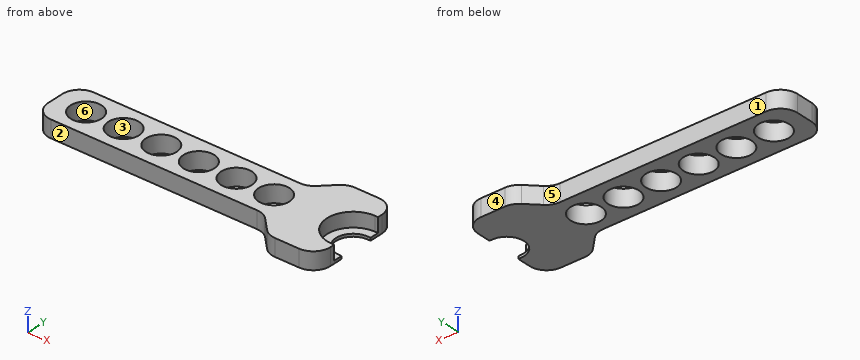
from build123d import *

# Parameters (mm, degrees)
F1_DEPTH    = 6.35
F3_DEPTH    = 5.334
F4_W        = 17.78
F4_H        = 8.255
F5_DEPTH    = 25.4
F6_R        = 5.715
F7_DEPTH    = 25.4
F8_T4_DEPTH = 6.35
F8_T9_DEPTH = 6.35
F9_R        = 6.35


# Not quite as in the source:
# - a fillet or chamfer that OpenCascade refuses, or shapes differently, is made with other operations: its cross-section is extruded or revolved along the edge and cut away or added


with BuildPart() as f1:
    # F0 (on Top) → F1 (new body)
    with BuildSketch(Plane.XY):
        Polygon((8.1444730278, -17.78), (17.78, -17.78), (17.78, 17.78), (-17.78, 17.78), (-17.78, 9.525), (-93.98, 9.525), (-93.98, -9.525), (-17.78, -9.525), (-17.78, -17.78), (-8.1444730278, -17.78), align=None)
    extrude(amount=F1_DEPTH)

    # F2 (on face) → F3 (cut)
    with BuildSketch(Plane.XY.offset(6.35)):
        with BuildLine():
            Line((17.78, 9.7409), (16.7259, 9.7409))
            ThreePointArc((16.7259, 9.7409), (6.985, 0), (16.7259, -9.7409))
            Line((16.7259, -9.7409), (17.78, -9.7409))
            Line((17.78, -9.7409), (17.78, 9.7409))
        make_face()
    extrude(amount=-F3_DEPTH, mode=Mode.SUBTRACT)

    # F4 (on face) → F5 (cut)
    with BuildSketch(Plane(origin=(0, 0, 0), x_dir=(1, 0, 0), z_dir=(0, 0, -1))):
        with BuildLine():
            Line((17.78, 6.4135), (16.7005, 6.4135))
            ThreePointArc((16.7005, 6.4135), (10.287, 0), (16.7005, -6.4135))
            Line((16.7005, -6.4135), (17.78, -6.4135))
            Line((17.78, -6.4135), (17.78, 6.4135))
        make_face()
        with Locations((-8.89, -13.6525)):
            Rectangle(F4_W, F4_H)
        with Locations((-8.89, 13.6525)):
            Rectangle(F4_W, F4_H)
    extrude(amount=-F5_DEPTH, mode=Mode.SUBTRACT)

    # F6 (on face) → F7 (cut)
    with BuildSketch(Plane.XY.offset(6.35)):
        with Locations((-82.55, 0)):
            Circle(F6_R)
        with Locations((-68.58, 0)):
            Circle(F6_R)
        with Locations((-54.61, 0)):
            Circle(F6_R)
        with Locations((-40.64, 0)):
            Circle(F6_R)
        with Locations((-26.67, 0)):
            Circle(F6_R)
        with Locations((-12.7, 0)):
            Circle(F6_R)
    extrude(amount=-F7_DEPTH, mode=Mode.SUBTRACT)

    # F8: chamfer of 8.382 on 2 edges, made by hand


with BuildPart() as f8_tool2:
    # F8_s3 → F8_t4 (new body)
    with BuildSketch(Plane.XY):
        Polygon((0, -17.907), (-8.382, -9.525), (0, -9.525), align=None)
    extrude(amount=F8_T4_DEPTH)

    split(bisect_by=Plane.XZ.offset(17.78), keep=Keep.BOTTOM)


with BuildPart() as f1_1:
    add(f1.part)

    # F8_t1: union F8_tool2
    add(f8_tool2.part)


with BuildPart() as f8_tool7:
    # F8_s8 → F8_t9 (new body)
    with BuildSketch(Plane.XY):
        Polygon((-8.382, 9.525), (0, 17.907), (0, 9.525), align=None)
    extrude(amount=F8_T9_DEPTH)

    split(bisect_by=Plane.XZ.offset(-17.78), keep=Keep.TOP)


with BuildPart() as f1_2:
    add(f1_1.part)

    # F8_t6: union F8_tool7
    add(f8_tool7.part)

    # F9
    f9_edges = [f1_2.edges().sort_by_distance(p)[0] for p in [
        (-8.382, -9.525, 3.175),
        (-8.382, 9.525, 3.175),
        (-0.127, 17.78, 3.175),
        (-0.127, -17.78, 3.175),
        (-93.98, 9.525, 3.175),
        (-93.98, -9.525, 3.175),
        (17.78, 17.78, 3.175),
        (17.78, -17.78, 3.175),
    ]]
    fillet(f9_edges, radius=F9_R)


solid = f1_2.part
Read the model definition and answer for the solid it produces. Units are mm, in the model's axes. Face numbers are marked on the shaded views. A direction names the side the tool comes from. Round coordinates to 2 decimals unless told otherwise and drop trailing zeros. Write each loop counter-clockwise with the first axis right and the second up, starting at its lowest first coordinate (ties: lowest second). Pieces come first, ordered by that corner, then holes.
Q1. Find section B-B on y = 0. State how many separate pieces and enclosed holes the cut face has, and give its area (3 significant figures).
Values:
separate pieces: 7
enclosed holes: 0
area: 209 mm2
Q2. The mould has two halves that part along X. Classify the marked faces 4, 5 and 6: released by +X, released by -X, zero draft, split by the parting line, or undercut.
Values:
face 4: zero draft
face 5: released by -X
face 6: undercut
Q3. Straight lines are drawn through the part: line 1 (Y direction, x = -82.55, z = 2.25) (3 decimals); line 2 (X direction, y = 11.5, z = 2); line 3 (Y direction, x = -39, z = 3) (3 decimals). For each, find the intervals that lie inside material, in ascending order.
Values:
line 1: y = -9.525 to -5.715, 5.715 to 9.525
line 2: x = -6.41 to 17.78
line 3: y = -9.525 to -5.475, 5.475 to 9.525
Q4. Find section A-A on x = -54.61. Determine the outline of the cut face in (y, z) (3 decimals), and give its area (3 significant figures).
Values:
outline: (-9.525, 0) - (-5.715, 0) - (-5.715, 6.35) - (-9.525, 6.35) - close; (5.715, 0) - (9.525, 0) - (9.525, 6.35) - (5.715, 6.35) - close
area: 48.4 mm2
Q5. Find section D-D on x = -69. Determine the outline of the cut face in (y, z) (3 decimals), and give its area (3 significant figures).
Values:
outline: (-9.525, 0) - (-5.7, 0) - (-5.7, 6.35) - (-9.525, 6.35) - close; (5.7, 0) - (9.525, 0) - (9.525, 6.35) - (5.7, 6.35) - close
area: 48.6 mm2
Q6. Find section C-C on z = 3. Determine the outline of the cut face in (x, y) (3 decimals), and give its area (3 significant figures).
Values:
outline: (-93.98, -3.175) arc R6.35 ccw to (-87.63, -9.525) - (-11.012, -9.525) arc R6.35 cw to (-6.522, -11.385) - (-1.987, -15.92) arc R6.35 ccw to (2.503, -17.78) - (11.43, -17.78) arc R6.35 ccw to (17.78, -11.43) - (17.78, -9.741) - (16.726, -9.741) arc R9.741 cw to (16.726, 9.741) - (17.78, 9.741) - (17.78, 11.43) arc R6.35 ccw to (11.43, 17.78) - (2.503, 17.78) arc R6.35 ccw to (-1.987, 15.92) - (-6.522, 11.385) arc R6.35 cw to (-11.012, 9.525) - (-87.63, 9.525) arc R6.35 ccw to (-93.98, 3.175) - close; hole circle Ø11.43 at (-82.55, 0); hole circle Ø11.43 at (-68.58, 0); hole circle Ø11.43 at (-54.61, 0); hole circle Ø11.43 at (-40.64, 0); hole circle Ø11.43 at (-26.67, 0); hole circle Ø11.43 at (-12.7, 0)
area: 1,670 mm2
Q7. Flat-ended cylindrical pins translate along their axes: P1, Ø3, axis at x = 14, y = -3.5, coming from the +Z side; P2, Ø0.5, axis at x = 17, z = 0.5, coming from the +Y side; P3, Ø0.8, axis at x = 17, z = 0.5, coming from the -Y side; P4, Ø0.8, axis at x = 17.5, z = 5, coming from the +Y side. Find the tip coordinate at first contact, or state that the pin passes through.
Values:
P1: passes through
P2: stops at y = 14.9
P3: stops at y = -15.12
P4: stops at y = 14.29
Q8. A tool of negligible diameter and unlimited length cuts with its end or side. For the marked faces 1, 2 and 3, from which of +Z, -Z, +X, -X, +Y, -Y can it reach the whole face along a straight path? Write none if from no direction.
Values:
face 1: +Z, -Z, -X, +Y
face 2: +Z, -Z, -X, -Y
face 3: +Z, -Z
